```python
from build123d import *

# Parameters (mm, degrees)
FILLET1_R     = 1
CHAMFER1_SIZE = 0.5


with BuildPart() as part:
    # Sketch1 → Revolve1 (revolve)
    with BuildSketch(Plane.XY, mode=Mode.PRIVATE) as revolve1_sk:
        Polygon((12.9, 5.5), (12.9, 3), (8.9, 3), (8.9, 0), (10.9, 0), (10.9, 1), (14.9, 1), (14.9, 5.5), align=None)
    revolve(revolve1_sk.sketch.rotate(Axis((0, 0, 0), (0, 1, 0)), 90), axis=Axis((0, 0, 0), (0, 1, 0)))

    # Fillet1
    fillet1_edges = [part.edges().sort_by_distance(p)[0] for p in [
        (0, 1, 14.9),
    ]]
    fillet(fillet1_edges, radius=FILLET1_R)

    # Chamfer1
    chamfer1_edges = [part.edges().sort_by_distance(p)[0] for p in [
        (0, 5.5, 12.9),
        (0, 3, 8.9),
    ]]
    chamfer(chamfer1_edges, length=CHAMFER1_SIZE)


solid = part.part
```
Design review of the part built by this model. Coordinates are the model's own, in mm. A direction names the side the tool comes from. Round coordinates to 2 decimals unless told otherwise and drop trailing zeros. Write each loop counter-clockwise with the first axis right and the second up, starting at its lowest first coordinate (ties: lowest second). Pieces come first, ordered by that corner, then holes. Notation, with made-up numbers: (59.25, 82) -> (111.25, 82) arc R21 cw to (111.25, 113) -> close; hole circle Ø3 at (60, -28.5). An arc over 180 degrees is marked (long way). Write item = value, one per line. Start each with the question number.
1) Take a section at B-B, the plane x = 0. State the section outline as (y, z) points.
2) Mouldability with a two-part tool opening along Z and no side actions: class faces 4 (the face through (11.445, 3.986, -5.953)), 5 (the face through (9.67, 0.51, -5.03)), 6 (the face through (9, 0, 2)) as +Z half, -Z half, draft (parallel to the pull), parting line (faces both ways), or undercut.
3) Tool access review of faces 1 (the face through (6.1, 1, -9.3)), 2 (the face through (8, 3, 6)), 3 (the face through (-6.015, 1.232, 6.56)): name each direction out of +Z, -Z, +X, -X, +Y, -Y from which nothing blocks a thin tool from reaching the whole face with its end or side.
4) Wall thickness on probe 1 along X at (y, z) = (2.05, 0); probe 2 along X at (y, z) = (4.3, 0); probe 3 along Y at (x, z) = (-12.25, 5.75): over which ranges is each line inside the solid? List them lowest first. Write a range as from..to.
5) Clearance check with flat-ended pins moving along their axes: pin 1 (13 mm diameter, centred on x = -4, z = -4.5, fed in from +Y); pin 2 (2 mm diameter, centred on x = 4.5, z = 4, fed in from +Y); pin 3 (2 mm diameter, centred on x = -4, y = 2, fed in from +Z); pin 4 (1.5 mm diameter, centred on x = -9.5, y = 4, fed in from -Z). State where each tip first meets the part, or that it passes through.
6) Take a section at A-A, the plane z = 0. State the section outline as (x, y) points.
7) Take a section at C-C, the plane y = 3.9. State the section outline as (x, z) points, plus the area to 3 significant figures.
Results list:
q1.outline = (0, -10.9) -> (1, -10.9) -> (1, -13.9) arc R1 ccw to (2, -14.9) -> (5.5, -14.9) -> (5.5, -13.4) -> (5, -12.9) -> (3, -12.9) -> (3, -9.4) -> (2.5, -8.9) -> (0, -8.9) -> close; (0, 8.9) -> (2.5, 8.9) -> (3, 9.4) -> (3, 12.9) -> (5, 12.9) -> (5.5, 13.4) -> (5.5, 14.9) -> (2, 14.9) arc R1 ccw to (1, 13.9) -> (1, 10.9) -> (0, 10.9) -> close
q2.face_4 = undercut
q2.face_5 = parting line
q2.face_6 = draft
q3.face_1 = -Y
q3.face_2 = +Y
q3.face_3 = +Y, -Y
q4.probe_1 = -14.9..-8.9, 8.9..14.9
q4.probe_2 = -14.9..-12.9, 12.9..14.9
q4.probe_3 = 1..5.5
q5.pin_1 = 3
q5.pin_2 = through
q5.pin_3 = 14.59
q5.pin_4 = -12.06
q6.outline = (-14.9, 2) arc R1 ccw to (-13.9, 1) -> (-10.9, 1) -> (-10.9, 0) -> (-8.9, 0) -> (-8.9, 2.5) -> (-9.4, 3) -> (-12.9, 3) -> (-12.9, 5) -> (-13.4, 5.5) -> (-14.9, 5.5) -> close; (8.9, 0) -> (10.9, 0) -> (10.9, 1) -> (13.9, 1) arc R1 ccw to (14.9, 2) -> (14.9, 5.5) -> (13.4, 5.5) -> (12.9, 5) -> (12.9, 3) -> (9.4, 3) -> (8.9, 2.5) -> close
q7.outline = circle Ø29.8 at (0, 0); hole circle Ø25.8 at (0, 0)
q7.area = 175 mm²
